from build123d import *

# Parameters (mm, degrees)
SKETCH_R        = 1.2
SKETCH_R_2      = 2.5
PAD_DEPTH       = 8.75
SKETCH001_R     = 8.25
POCKET_DEPTH    = 15
POCKET001_DEPTH = 3
SKETCH003_R     = 1.75
POCKET002_DEPTH = 6.001
CHAMFER_SIZE    = 0.75


with BuildPart() as part:
    # Sketch → Pad (new body, symmetric)
    with BuildSketch(Plane.YZ):
        with BuildLine():
            Line((-22, 14.25), (22, 14.25))
            Line((22, 14.25), (22, 8.25))
            Line((22, 8.25), (14, 8.25))
            ThreePointArc((14, 8.25), (11.87868, 7.37132), (11, 5.25))
            Line((11, 5.25), (11, 0))
            ThreePointArc((-11, 0), (0, -11), (11, 0))
            Line((-11, 0), (-11, 5.25))
            ThreePointArc((-11, 5.25), (-11.87868, 7.37132), (-14, 8.25))
            Line((-14, 8.25), (-22, 8.25))
            Line((-22, 8.25), (-22, 14.25))
        make_face()
        with Locations((-4.5, 0)):
            Circle(SKETCH_R, mode=Mode.SUBTRACT)
        with Locations((4.5, 0)):
            Circle(SKETCH_R, mode=Mode.SUBTRACT)
        Circle(SKETCH_R_2, mode=Mode.SUBTRACT)
    extrude(amount=PAD_DEPTH, both=True)

    # Sketch001 (on Face14 of Pad) → Pocket (cut)
    with BuildSketch(Plane(origin=(-8.75, 0, 0), x_dir=(0, 1, 0), z_dir=(-1, 0, 0))):
        Circle(SKETCH001_R)
    extrude(amount=-POCKET_DEPTH, mode=Mode.SUBTRACT)

    # Sketch002 (on Face7 of Pocket) → Pocket001 (cut)
    with BuildSketch(Plane.YX.offset(-8.25)):
        Polygon((-15.825684, 7.4), (-19.174316, 7.4), (-20.848632, 4.5), (-19.174316, 1.6), (-15.825684, 1.6), (-14.151368, 4.5), align=None)
        Polygon((-14.151368, -4.5), (-15.825684, -1.6), (-19.174316, -1.6), (-20.848632, -4.5), (-19.174316, -7.4), (-15.825684, -7.4), align=None)
        Polygon((19.174316, 1.6), (20.848632, 4.5), (19.174316, 7.4), (15.825684, 7.4), (14.151368, 4.5), (15.825684, 1.6), align=None)
        Polygon((19.174316, -7.4), (20.848632, -4.5), (19.174316, -1.6), (15.825684, -1.6), (14.151368, -4.5), (15.825684, -7.4), align=None)
    extrude(amount=-POCKET001_DEPTH, mode=Mode.SUBTRACT)

    # Sketch003 (on Face7 of Pocket001) → Pocket002 (cut, through all)
    with BuildSketch(Plane.YX.offset(-8.25)):
        with Locations((-17.5, 4.5)):
            Circle(SKETCH003_R)
        with Locations((-17.5, -4.5)):
            Circle(SKETCH003_R)
        with Locations((17.5, -4.5)):
            Circle(SKETCH003_R)
        with Locations((17.5, 4.5)):
            Circle(SKETCH003_R)
    extrude(amount=-POCKET002_DEPTH, mode=Mode.SUBTRACT)

    # Chamfer
    chamfer_edges = [part.edges().sort_by_distance(p)[0] for p in [
        (8.75, 3.3, 0),
        (8.75, -5.7, 0),
    ]]
    chamfer(chamfer_edges, length=CHAMFER_SIZE)


solid = part.part
Work out the finished part from the listing and answer in its coordinate system (mm). A direction names the side the tool comes from. Give positions to 0.01 mm unless a question says otherwise; leave off trailing zeros. Loops run counter-clockwise (first coordinate to the right, second up) from the corner with the lowest first, then second, coordinate; pieces in that order, holes last. Notation, with made-up numbers: (7.5, -3.5) - (32.5, -3.5) arc R11 cw to (32.5, 7.5) - close; hole circle Ø5 at (8.5, 63.5). An arc over 180 degrees is marked (long way). Answer in a Markdown table with one row per item. Add a question column.
Q1. Each of these flat-tipped pins is pushed along its axis until it touches: P1, Ø3, axis at y = -4.5, z = 0, coming from the +X side; P2, Ø2, axis at x = -4.5, y = 17.5, coming from the -Z side; P3, Ø10, axis at x = 1.5, z = -7, coming from the +Y side; P4, Ø8, axis at x = -1, z = -8, coming from the -Y side. Where does it stop, or does it pass through?
Q2. Determine the mould class of faces 4 (the cylindrical face through (0, 0, -11)), 5 (the flat face through (-5.97, -15, 9.73)), 6 (the cylindrical face through (7.48, -0.54, -2.44)) for opening direction Z: released by +Z, released by -Z, zero draft, split by the parting line, or undercut.
Q3. The part is cut by section C-C (y = 0). Determine the outline of the cut face in (x, z).
Q4. The part is cut by section B-B (x = 1). Determine the outline of the cut face in (y, z), and give its area (3 significant figures).
Q5. The part is cut by section D-D (z = 6). Determine the outline of the cut face in (x, y).
Q6. Consider line 1 along X through (y, z) = (-17.5, 12.6); line 2 along Z through (x, y) = (7.4, 0); line 3 along X through (y, z) = (-6.5, 5). Determine where each line is inside the solid, lowest interval first.
Q7. The part is cut by section A-A (y = 17.5). Determine the outline of the cut face in (x, z), and give its area (3 significant figures).
Q8. A tool of negligible diameter and unlimited length cuts with its end or side. For faces 1 (the flat face through (0, 11, 3)), 2 (the flat face through (-3.03, 15, 9.73)), 3 (the flat face through (0, -11, 3)), from which of +Z, -Z, +X, -X, +Y, -Y can it reach the whole face along a straight path? Write none if from no direction.
Solution:
| question | item | result |
|---|---|---|
| 1 | P1 | stops at x = 8.3 |
| 1 | P2 | passes through |
| 1 | P3 | stops at y = 10.82 |
| 1 | P4 | stops at y = -10.25 |
| 2 | face 4 | released by -Z |
| 2 | face 5 | zero draft |
| 2 | face 6 | undercut |
| 3 | outline | (-8.75, -11) - (8.75, -11) - (8.75, -2.5) - (6.25, -2.5) - (6.25, -8.25) - (-8.75, -8.25) - close; (-8.75, 8.25) - (6.25, 8.25) - (6.25, 2.5) - (8.75, 2.5) - (8.75, 14.25) - (-8.75, 14.25) - close |
| 4 | outline | (-22, 8.25) - (-14, 8.25) arc R3 cw to (-11, 5.25) - (-11, 0) arc R11 ccw to (11, 0) - (11, 5.25) arc R3 cw to (14, 8.25) - (22, 8.25) - (22, 14.25) - (-22, 14.25) - close; hole circle Ø16.5 at (0, 0) |
| 4 | area | 426 mm² |
| 5 | outline | (-8.75, -11.1) - (8.75, -11.1) - (8.75, 11.1) - (-8.75, 11.1) - (-8.75, 5.66) - (6.25, 5.66) - (6.25, -5.66) - (-8.75, -5.66) - close |
| 6 | line 1 | x = -8.75 to -6.25, -2.75 to 2.75, 6.25 to 8.75 |
| 6 | line 2 | z = -11 to -2.5, 2.5 to 14.25 |
| 6 | line 3 | x = 6.25 to 8.75 |
| 7 | outline | (-8.75, 8.25) - (-7.4, 8.25) - (-7.4, 11.25) - (-6.25, 11.25) - (-6.25, 14.25) - (-8.75, 14.25) - close; (-2.75, 11.25) - (-1.6, 11.25) - (-1.6, 8.25) - (1.6, 8.25) - (1.6, 11.25) - (2.75, 11.25) - (2.75, 14.25) - (-2.75, 14.25) - close; (6.25, 11.25) - (7.4, 11.25) - (7.4, 8.25) - (8.75, 8.25) - (8.75, 14.25) - (6.25, 14.25) - close |
| 7 | area | 49.2 mm² |
| 8 | face 1 | -Z, +X, -X, +Y |
| 8 | face 2 | -Z |
| 8 | face 3 | -Z, +X, -X, -Y |
